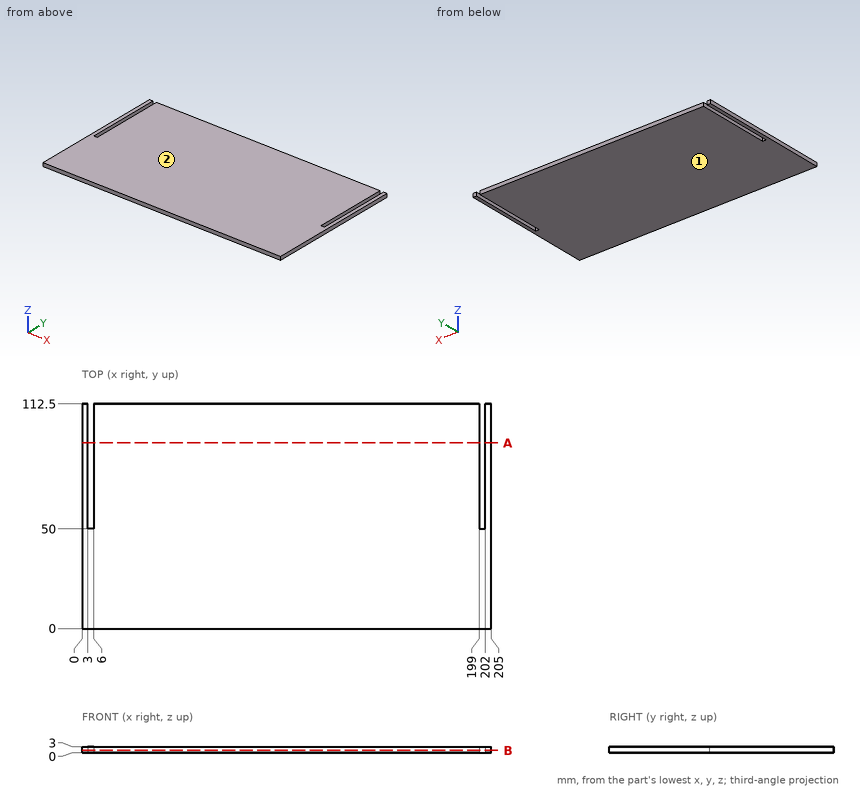
Here's the drawing with two shaded views (mm, measured from the low corner). I have some questions. Give positions to 0.01 mm unless a question says otherwise; leave off trailing zeros. Write each loop counter-clockwise with the first axis right and the second up, starting at its lowest first coordinate (ties: lowest second). Pieces come first, ordered by that corner, then holes. Notation, with made-up numbers: (72.25, 1) -> (91.25, 1) arc R19 ccw to (91.25, 7) -> close; hole circle Ø5 at (64, 47.25). An arc over 180 degrees is marked (long way). Use one line per item in the form item = value. Start each with the question number.
1. If I drill on L1, parallel to X at y = 96, z = 1.8, over which ranges is the centre line in solid material (lowest first)?
2. Imagine slicing it at A-A on y = 93. List the corners of the cut face in (x, z) for me, plus the area to 3 significant figures.
3. Thinking about a two-plate mould opening in Z: for the marked faces 1 and 2, which applies, +Z half, -Z half, draft (parallel to the pull), parting line (faces both ways), or undercut?
4. Imagine slicing it at B-B on z = 1.1. List the corners of the cut face in (x, y) for me, plus the area to 3 significant figures.
Entries:
q1.L1 = 0 to 3, 6 to 199, 202 to 205
q2.outline = (0, 0) -> (3, 0) -> (3, 3) -> (0, 3) -> close; (6, 0) -> (199, 0) -> (199, 3) -> (6, 3) -> close; (202, 0) -> (205, 0) -> (205, 3) -> (202, 3) -> close
q2.area = 597 mm²
q3.face_1 = -Z half
q3.face_2 = +Z half
q4.outline = (0, 0) -> (205, 0) -> (205, 112.5) -> (202, 112.5) -> (202, 50) -> (199, 50) -> (199, 112.5) -> (6, 112.5) -> (6, 50) -> (3, 50) -> (3, 112.5) -> (0, 112.5) -> close
q4.area = 22,700 mm²
